Check sheet for the modelled part. Datum: model origin and axes. Units: mm. Round coordinates to 2 decimals unless told otherwise and drop trailing zeros. Order: outer loops, then holes, each group sorted by start corner. A loop starts at its lowest first (then second) coordinate and runs counter-clockwise, first axis right, second up. Notation, with made-up numbers: (-11.5, -25.75) -> (45.5, -25.75) arc R14 ccw to (45.5, -17.75) -> close; hole circle Ø1 at (62, 2.25). An arc over 180 degrees is marked (long way). Answer in a Markdown table with one row per item.
Autodesk Inventor part; units mm, degrees
ref_plane "YZ Plane" through (0, 0, 0) normal (1, 0, 0) x (0, 1, 0)
ref_plane "XZ Plane" through (0, 0, 0) normal (0, 1, 0) x (-1, 0, 0)
ref_plane "XY Plane" through (0, 0, 0) normal (0, 0, 1) x (1, 0, 0)
sketch "Sketch1" plane through (0, 0, 0) normal (0, 0, 1) x (1, 0, 0)
  line L0 (0, 0) -> (120, 0)
  line L1 (120, 0) -> (120, 80)
  line L2 (120, 80) -> (0, 80)
  line L3 (0, 80) -> (0, 0)
  dimension "d0" = 120
  dimension "d1" = 80
extrude "Extrusion1" add sketch "Sketch1" along normal blind 6
sketch "Sketch2" plane through (0, 0, 6) normal (0, 0, 1) x (1, 0, 0)
  line L0 (0, 0) -> (120, 0)
  line L1 (120, 0) -> (120, 80)
  line L2 (120, 80) -> (0, 80)
  line L3 (0, 80) -> (0, 0)
  line L4 (0, 80) -> (14.75, 80)
  line L5 (14.75, 80) -> (14.75, 74)
  line L6 (14.75, 74) -> (0, 74)
  line L7 (0, 74) -> (0, 80)
  line L8 (120, 80) -> (0, 80)
  line L9 (45.25, 80) -> (74.75, 80)
  line L10 (74.75, 80) -> (74.75, 74)
  line L11 (74.75, 74) -> (45.25, 74)
  line L12 (45.25, 74) -> (45.25, 80)
  line L13 (120, 80) -> (105.25, 80)
  line L14 (105.25, 80) -> (105.25, 74)
  line L15 (105.25, 74) -> (120, 74)
  line L16 (120, 74) -> (120, 80)
  line L17 (120, 0) -> (105.25, 0)
  line L18 (105.25, 0) -> (105.25, 6)
  line L19 (105.25, 6) -> (120, 6)
  line L20 (120, 6) -> (120, 0)
  line L21 (0, 0) -> (120, 0)
  line L22 (74.75, 0) -> (45.25, 0)
  line L23 (45.25, 0) -> (45.25, 6)
  line L24 (45.25, 6) -> (74.75, 6)
  line L25 (74.75, 6) -> (74.75, 0)
  line L26 (0, 0) -> (14.75, 0)
  line L27 (14.75, 0) -> (14.75, 6)
  line L28 (14.75, 6) -> (0, 6)
  line L29 (0, 6) -> (0, 0)
  line L30 (60, 104.1502) -> (60, -33.6862)
  line L31 (120, 0) -> (120, 80)
  dimension "d4" = 6
  dimension "d5" = 6
  dimension "d6" = 14.75
  dimension "d7" = 29.5
  dimension "d9" = 14.75
  dimension "d19" = 60
  dimension "d20" = 14.75
extrude "Extrusion2" cut sketch "Sketch2" against normal up to next contours L3 L28 L27 L0 | L23 L24 L30 L0 | L3 L2 L5 L6 | L30 L24 L25 L0 | L18 L19 L1 L0 | L30 L2 L10 L11 | L11 L12 L2 L30 | L15 L14 L2 L1
sketch "Sketch4" plane through (0, 0, 6) normal (0, 0, 1) x (1, 0, 0)
  circle A0 centre (40, 40) radius 4.6
  line L0 (0, 74) -> (0, 6)
  line L1 (45.25, 80) -> (14.75, 80)
  point P0 (0, 0)
  dimension "d14" = 40
  dimension "d15" = 40
  dimension "d16" = 9.2
extrude "Extrusion4" cut sketch "Sketch4" against normal up to next
sketch "Sketch5" plane through (0, 0, 6) normal (0, 0, 1) x (1, 0, 0)
  circle A0 centre (40, 40) radius 4.6
  line L0 (74.75, 6) -> (74.75, 0)
  line L1 (74.75, 0) -> (105.25, 0)
  line L2 (105.25, 0) -> (105.25, 6)
  line L3 (105.25, 6) -> (120, 6)
  line L4 (120, 6) -> (120, 74)
  line L5 (120, 74) -> (105.25, 74)
  line L6 (105.25, 74) -> (105.25, 80)
  line L7 (105.25, 80) -> (74.75, 80)
  line L8 (74.75, 80) -> (74.75, 74)
  line L9 (74.75, 74) -> (45.25, 74)
  line L10 (45.25, 74) -> (45.25, 80)
  line L11 (45.25, 80) -> (14.75, 80)
  line L12 (14.75, 80) -> (14.75, 74)
  line L13 (14.75, 74) -> (0, 74)
  line L14 (0, 74) -> (0, 6)
  line L15 (0, 6) -> (14.75, 6)
  line L16 (14.75, 6) -> (14.75, 0)
  line L17 (14.75, 0) -> (45.25, 0)
  line L18 (45.25, 0) -> (45.25, 6)
  line L19 (45.25, 6) -> (74.75, 6)
  line L20 (52.5, 27.5) -> (27.5, 27.5)
  line L21 (27.5, 27.5) -> (27.5, 52.5)
  line L22 (27.5, 52.5) -> (52.5, 52.5)
  line L23 (52.5, 52.5) -> (52.5, 27.5)
  circle A1 centre (40, 40) radius 14.125
  circle A2 centre (52.5, 27.5) radius 1.5
  circle A3 centre (27.5, 27.5) radius 1.5
  circle A4 centre (27.5, 52.5) radius 1.5
  circle A5 centre (52.5, 52.5) radius 1.5
  circle A6 centre (40, 40) radius 26.387 construction
  line L24 (40, 40) -> (40, 13.613) construction
  line L25 (40, 40) -> (17.1482, 26.8065) construction
  arc A7 (40, 11.613) -> (40, 15.613) centre (40, 13.613) ccw
  arc A8 (18.8802, 27.8065) -> (15.4161, 25.8065) centre (17.1482, 26.8065) ccw
  arc A9 (18.8802, 27.8065) -> (40, 15.613) centre (40, 40) ccw
  arc A10 (15.4161, 25.8065) -> (40, 11.613) centre (40, 40) ccw
  point P0 (0, 0)
  dimension "d21" = 3
  dimension "d22" = 3
  dimension "d23" = 3
  dimension "d24" = 3
  dimension "d25" = 28.25
  dimension "d26" = 25
  dimension "d27" = 25
  dimension "d28" = 12.5
  dimension "d29" = 12.5
  dimension "d30" = 52.774
  dimension "d31" = 60
  dimension "d32" = 4
  dimension "d33" = 4
extrude "Extrusion5" cut sketch "Sketch5" against normal blind 10 contours A3 L21 L20 | L20 L21 A3 | A1 L21 L22 L23 L20 | L20 A1 | A1 L21 | A2 L23 L20 | L20 L23 A2 | L23 A1 | A4 L22 L21 | L21 L22 A4 | A1 L22 | A5 L22 L23 | L23 L22 A5 | A10 A8 A9 A7
equation "\"d20\" = 0.5 * d7"
equation "\"d22\" = d21"
equation "\"d23\" = d21"
equation "\"d24\" = d21"
equation "\"d28\" = 0.5 * d26"
equation "\"d29\" = 0.5 * d27"
properties part number "top"
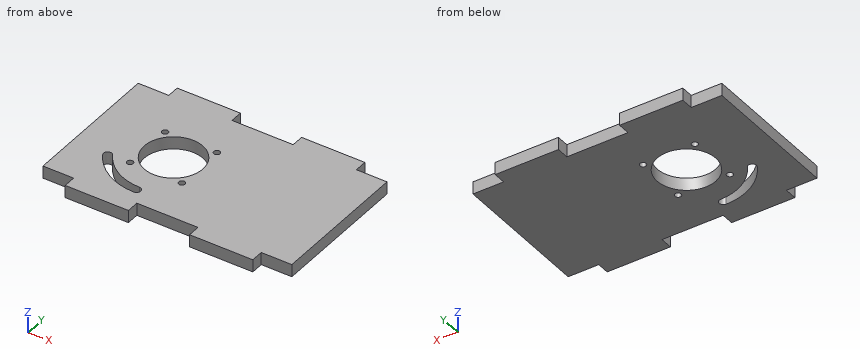
(1) Scan lines: probe 1 along Y at (x, z) = (40, 4.75) (3 decimals); probe 2 along Y at (x, z) = (32.5, 3.45); probe 3 along X at (y, z) = (39.5, 3). Record each from-to range of solid material in increasing order. Write a range as from..to.
Solutions:
| item | result |
|---|---|
| probe 1 | 0..11.613, 15.613..25.875, 54.125..80 |
| probe 2 | 0..12.62, 16.79..28.03, 51.97..80 |
| probe 3 | 0..25.88, 54.12..120 |
(2) Depth check by flat-ended pin: pin 1 Ø1.8 at (y, z) = (1.5, 3) entering from +X; pin 2 Ø1.8 at (x, y) = (27.5, 27.5) entering from +Z; pin 3 Ø3 at (x, z) = (5.5, 2.5) entering from -Y; pin 4 Ø3 at (x, y) = (60, 65.5) entering from -Z. Enter the tip coordinate at first touch or a pass-through.
Solutions:
| item | result |
|---|---|
| pin 1 | x = 105.25 |
| pin 2 | through |
| pin 3 | y = 6 |
| pin 4 | z = 0 |
(3) Section check C-C on z = 1.25. Give the number of separate pieces and of enclosed holes in the cut face, plus the area to 3 significant figures.
Solutions:
| item | result |
|---|---|
| separate pieces | 1 |
| enclosed holes | 6 |
| area | 8,110 mm^2 |
(4) Section check D-D on x = 27.5. Record the boundary of the cut face in (y, z), plus the area to 3 significant figures.
Solutions:
| item | result |
|---|---|
| outline | (0, 0) -> (14.51, 0) -> (14.51, 6) -> (0, 6) -> close; (19.06, 0) -> (26, 0) -> (26, 6) -> (19.06, 6) -> close; (29, 0) -> (33.42, 0) -> (33.42, 6) -> (29, 6) -> close; (46.58, 0) -> (51, 0) -> (51, 6) -> (46.58, 6) -> close; (54, 0) -> (80, 0) -> (80, 6) -> (54, 6) -> close |
| area | 338 mm^2 |
(5) Section check A-A on y = 40. Record the boundary of the cut face in (x, z) (3 decimals).
Solutions:
| item | result |
|---|---|
| outline | (0, 0) -> (25.875, 0) -> (25.875, 6) -> (0, 6) -> close; (54.125, 0) -> (120, 0) -> (120, 6) -> (54.125, 6) -> close |
(6) Section check B-B on y = 52.5. Record the boundary of the cut face in (x, z), plus the area to 3 significant figures.
Solutions:
| item | result |
|---|---|
| outline | (0, 0) -> (26, 0) -> (26, 6) -> (0, 6) -> close; (29, 0) -> (33.42, 0) -> (33.42, 6) -> (29, 6) -> close; (46.58, 0) -> (51, 0) -> (51, 6) -> (46.58, 6) -> close; (54, 0) -> (120, 0) -> (120, 6) -> (54, 6) -> close |
| area | 605 mm^2 |
